from build123d import *

# Parameters (mm, degrees)
F0_W     = 25.4
F0_H     = 50.8
F0_W_2   = 19.05
F0_H_2   = 44.45
F1_DEPTH = 304.8
F2_R     = 2.5527
F3_DEPTH = 50.801
F5_DEPTH = 25.401


with BuildPart() as f1:
    # F0 (on Front) → F1 (new body, symmetric)
    with BuildSketch(Plane.XZ):
        with Locations((12.7, 25.4)):
            Rectangle(F0_W, F0_H)
        with Locations((12.7, 25.4)):
            Rectangle(F0_W_2, F0_H_2, mode=Mode.SUBTRACT)
    extrude(amount=F1_DEPTH, both=True)

    # F2 (on face) → F3 (cut, through all)
    with BuildSketch(Plane.XY.offset(50.8)):
        with BuildLine():
            ThreePointArc((12.7, 294.6527), (10.8949685197, 290.2949685197), (15.2527, 292.1))
            ThreePointArc((15.2527, 292.1), (14.5050314803, 293.9050314803), (12.7, 294.6527))
        make_face()
        with Locations((12.7, 279.4)):
            Circle(F2_R)
        with Locations((12.7, 266.7)):
            Circle(F2_R)
        with Locations((12.7, 254)):
            Circle(F2_R)
        with Locations((12.7, 241.3)):
            Circle(F2_R)
        with Locations((12.7, 228.6)):
            Circle(F2_R)
        with Locations((12.7, 215.9)):
            Circle(F2_R)
        with Locations((12.7, 203.2)):
            Circle(F2_R)
        with Locations((12.7, 190.5)):
            Circle(F2_R)
        with Locations((12.7, 177.8)):
            Circle(F2_R)
        with Locations((12.7, 165.1)):
            Circle(F2_R)
        with Locations((12.7, 152.4)):
            Circle(F2_R)
        with Locations((12.7, 139.7)):
            Circle(F2_R)
        with Locations((12.7, 127)):
            Circle(F2_R)
        with Locations((12.7, 114.3)):
            Circle(F2_R)
        with Locations((12.7, 101.6)):
            Circle(F2_R)
        with Locations((12.7, 88.9)):
            Circle(F2_R)
        with Locations((12.7, 76.2)):
            Circle(F2_R)
        with Locations((12.7, 63.5)):
            Circle(F2_R)
        with Locations((12.7, 50.8)):
            Circle(F2_R)
        with Locations((12.7, 38.1)):
            Circle(F2_R)
        with Locations((12.7, 25.4)):
            Circle(F2_R)
        with Locations((12.7, 12.7)):
            Circle(F2_R)
        with Locations((12.7, 0)):
            Circle(F2_R)
        with Locations((12.7, -12.7)):
            Circle(F2_R)
        with Locations((12.7, -25.4)):
            Circle(F2_R)
        with Locations((12.7, -38.1)):
            Circle(F2_R)
        with Locations((12.7, -50.8)):
            Circle(F2_R)
        with Locations((12.7, -63.5)):
            Circle(F2_R)
        with Locations((12.7, -76.2)):
            Circle(F2_R)
        with Locations((12.7, -88.9)):
            Circle(F2_R)
        with Locations((12.7, -101.6)):
            Circle(F2_R)
        with Locations((12.7, -114.3)):
            Circle(F2_R)
        with Locations((12.7, -127)):
            Circle(F2_R)
        with Locations((12.7, -139.7)):
            Circle(F2_R)
        with Locations((12.7, -152.4)):
            Circle(F2_R)
        with Locations((12.7, -165.1)):
            Circle(F2_R)
        with Locations((12.7, -177.8)):
            Circle(F2_R)
        with Locations((12.7, -190.5)):
            Circle(F2_R)
        with Locations((12.7, -203.2)):
            Circle(F2_R)
        with Locations((12.7, -215.9)):
            Circle(F2_R)
        with Locations((12.7, -228.6)):
            Circle(F2_R)
        with Locations((12.7, -241.3)):
            Circle(F2_R)
        with Locations((12.7, -254)):
            Circle(F2_R)
        with Locations((12.7, -266.7)):
            Circle(F2_R)
        with Locations((12.7, -279.4)):
            Circle(F2_R)
        with Locations((12.7, -292.1)):
            Circle(F2_R)
    extrude(amount=-F3_DEPTH, mode=Mode.SUBTRACT)

    # F4 (on face) → F5 (cut, through all)
    with BuildSketch(Plane.YZ.offset(25.4)):
        with BuildLine():
            ThreePointArc((-247.65, 27.94), (-260.3490284744, 28.0510739923), (-247.6538858053, 27.7178860032))
            ThreePointArc((-247.6538858053, 27.7178860032), (-247.6509715256, 27.8289260077), (-247.65, 27.94))
        make_face()
        with BuildLine():
            Line((6.3461141947, 19.2721139968), (0, 19.05))
            Line((0, 19.05), (-6.3461141947, 19.2721139968))
            ThreePointArc((-6.3461141947, 19.2721139968), (-0.1110739923, 12.7009715256), (6.35, 19.05))
            ThreePointArc((6.35, 19.05), (6.3490284744, 19.1610739923), (6.3461141947, 19.2721139968))
        make_face()
        with BuildLine():
            Line((0, 25.4), (0, 19.05))
            Line((0, 19.05), (6.3461141947, 19.2721139968))
            ThreePointArc((6.3461141947, 19.2721139968), (4.410899915, 23.6179822613), (0, 25.4))
        make_face()
        with BuildLine():
            Line((-6.3461141947, 19.2721139968), (0, 19.05))
            Line((0, 19.05), (0, 25.4))
            ThreePointArc((0, 25.4), (-4.410899915, 23.6179822613), (-6.3461141947, 19.2721139968))
        make_face()
        with BuildLine():
            ThreePointArc((260.35, 27.94), (253.8889260077, 34.2890284744), (247.6538858053, 27.7178860032))
            ThreePointArc((247.6538858053, 27.7178860032), (254.1110739923, 21.5909715256), (260.35, 27.94))
        make_face()
    extrude(amount=-F5_DEPTH, mode=Mode.SUBTRACT)


solid = f1.part
Check sheet for the modelled part. Datum: model origin and axes. Units: mm. A direction names the side the tool comes from. Round coordinates to 2 decimals unless told otherwise and drop trailing zeros. Loops run counter-clockwise (first coordinate to the right, second up) from the corner with the lowest first, then second, coordinate; pieces in that order, holes last. Notation, with made-up numbers: (40.5, -3) -> (81.5, -3) arc R24 cw to (81.5, 14) -> close; hole circle Ø6 at (56.25, -38). An arc over 180 degrees is marked (long way). Put each result on its own line as item: value. Start each with the question number.
1. Access from +Z, -Z, +X, -X, +Y, -Y to the whole of each face (thin tool, end or side, straight path). Record for faces 1 (the face through (13, -4, 3.175)), 2 (the face through (25.4, -4, 25)).
2. Gauge pin test, flat end, axial feed: pin 1 (10 mm diameter, centred on x = 12.5, z = 9, fed in from -Y). Record the tip position at first contact, or that the pin passes through.
3. Scan lines: probe 1 along Z at (x, y) = (4.5, 246) (3 decimals); probe 2 along X at (y, z) = (129.5, 14) (3 decimals); probe 3 along X at (y, z) = (-215.9, 49.9). Record each from-to range of solid material in increasing order.
4. Section check A-A (z = 40). Enter the section's corners in (x, y) (3 decimals).
5. Draft check along X on faces 3 (the face through (0, -4, 25)), 4 (the face through (2, -304.8, 24)), 5 (the face through (13, -4, 47.625)). Enter one of: +X half, -X half, draft (parallel to the pull), parting line (faces both ways), or undercut.
Findings:
1. face 1: +Y, -Y
1. face 2: +Z, -Z, +X, +Y, -Y
2. pin 1: passes through
3. probe 1: z = 0 to 3.175, 47.625 to 50.8
3. probe 2: x = 0 to 3.175, 22.225 to 25.4
3. probe 3: x = 0 to 10.15, 15.25 to 25.4
4. outline: (0, -304.8) -> (3.175, -304.8) -> (3.175, 304.8) -> (0, 304.8) -> close; (22.225, -304.8) -> (25.4, -304.8) -> (25.4, 304.8) -> (22.225, 304.8) -> close
5. face 3: -X half
5. face 4: draft
5. face 5: undercut
